Design review of the part shown in the three views and the two pictorial views. Dimensions are in mm from the part's minimum x, y and z. A direction names the side the tool comes from. Coordinates: 2 decimals unless noted, no trailing zeros. Loops run counter-clockwise (first coordinate to the right, second up) from the corner with the lowest first, then second, coordinate; pieces in that order, holes last. Notation, with made-up numbers: M -23,78 L 31,78 A27 ccw 31,113 Z; hole C 13,-23.5 d11. An arc over 180 degrees is marked long. Use one line per item in the form item = value.
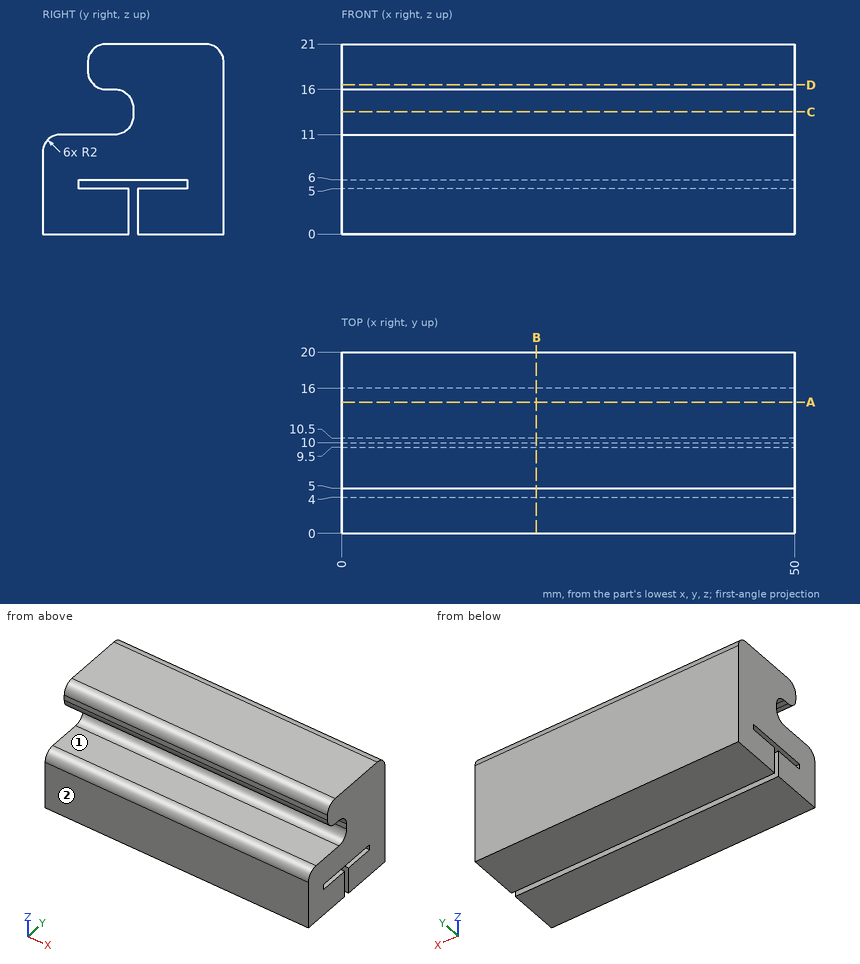
1. Machinability: for the marked faces 1 and 2, which of the approach directions +Z, -Z, +X, -X, +Y, -Y give a long, thin tool a straight path to every point of the face, cutting with its end or side? Answer none if there is none.
Response values:
face_1 = +X, -X, -Y
face_2 = +Z, -Z, +X, -X, -Y
2. Add section A-A (y = 14.5). State the section outline as (x, z) points, then the cut area to 3 significant figures.
Response values:
outline = M 0,0 L 50,0 L 50,5 L 0,5 Z; M 0,6 L 50,6 L 50,21 L 0,21 Z
area = 1,000 mm^2
3. Add section D-D (z = 16.5). State the section outline as (x, y) points, then the cut area to 3 significant figures.
Response values:
outline = M 0,5.68 L 50,5.68 L 50,20 L 0,20 Z
area = 716 mm^2
4. Add section C-C (z = 13.5). State the section outline as (x, y) points, then the cut area to 3 significant figures.
Response values:
outline = M 0,10 L 50,10 L 50,20 L 0,20 Z
area = 500 mm^2
5. Wall thickness on line 1 along Y through (x, z) = (28.5, 1.5); line 2 along Y through (x, z) = (7.5, 5.25); line 3 along Y through (x, z) = (38, 13.5): over which ranges is each line inside the solid? List them lowest first. Write a range as from..to.
Response values:
line_1 = 0..9.5, 10.5..20
line_2 = 0..4, 16..20
line_3 = 10..20
6. Insertion check: P1, Ø0.8, axis at x = 13.5, z = 13.5, coming from the -Y side; P2, Ø0.8, axis at x = 24.5, z = 18.5, coming from the -Y side; P3, Ø1.8, axis at x = 15.5, y = 5, coming from the +Z side. Each pin has a flat end and moves straight along its axis. Give the tip position at first contact, or say it passes through.
Response values:
P1 = 10
P2 = 5
P3 = 20.67
7. Add section B-B (x = 21.5). State the section outline as (y, z) points, then the cut area to 3 significant figures.
Response values:
outline = M 0,0 L 9.5,0 L 9.5,5 L 4,5 L 4,6 L 16,6 L 16,5 L 10.5,5 L 10.5,0 L 20,0 L 20,19 A2 ccw 18,21 L 7,21 A2 ccw 5,19 L 5,18 A2 ccw 7,16 L 8,16 A2 cw 10,14 L 10,13 A2 cw 8,11 L 2,11 A2 ccw 0,9 Z
area = 326 mm^2
